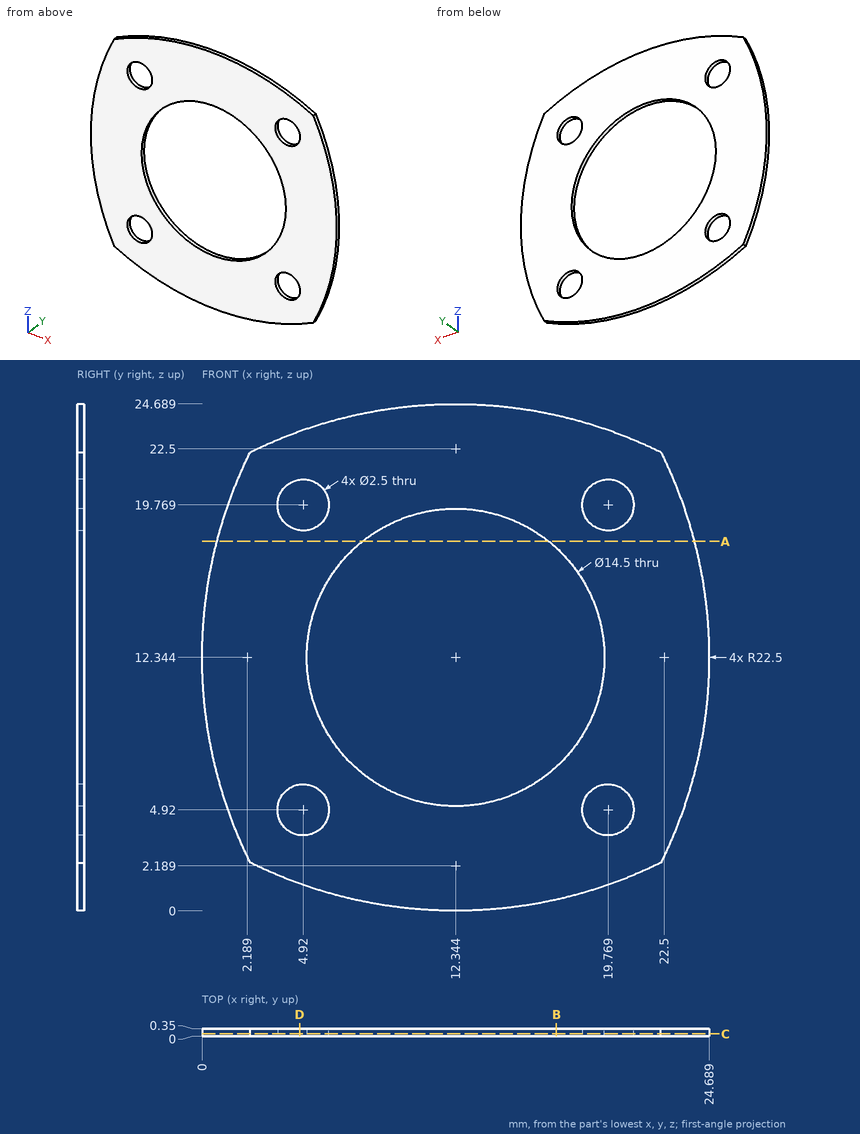
The figure shows three views and two pictorial views of one solid part (mm, origin at its lowest corner). Answer the questions. Round coordinates to 2 decimals unless told otherwise and drop trailing zeros. Write each loop counter-clockwise with the first axis right and the second up, starting at its lowest first coordinate (ties: lowest second). Pieces come first, ordered by that corner, then holes. Notation, with made-up numbers: (-28, -16) - (2, -16) arc R16 ccw to (2, 8) - close; hole circle Ø6 at (25, 82.25). An arc over 180 degrees is marked (long way). Answer in a Markdown table with one row per item. Add a question column.
1. Find the intervals of material crossed by line 1 along X through (y, z) = (0.25, 4) (1 decimal); line 2 along Z through (x, y) = (4.25, 0.15) (1 decimal), in increasing order. Write a range as from..to.
2. A cutting plane is placed at B-B, the plane x = 17.25. Determine the outline of the cut face in (y, z).
3. A cutting plane is placed at A-A, the plane z = 18. Determine the outline of the cut face in (x, y).
4. A cutting plane is placed at D-D, the plane x = 4.75. Determine the outline of the cut face in (y, z).
5. A cutting plane is placed at C-C, the plane y = 0.1. Count the separate pieces of the cut face and the enclosed holes in it, and give its area (3 significant figures).
Worked out:
| question | item | result |
|---|---|---|
| 1 | line 1 | 1.6..4.1, 5.8..18.9, 20.6..23.1 |
| 1 | line 2 | 1.5..3.9, 6..18.7, 20.8..23.2 |
| 2 | outline | (0, 0.54) - (0.35, 0.54) - (0.35, 7.01) - (0, 7.01) - close; (0, 17.68) - (0.35, 17.68) - (0.35, 24.15) - (0, 24.15) - close |
| 3 | outline | (0.72, 0) - (7.81, 0) - (7.81, 0.35) - (0.72, 0.35) - close; (16.88, 0) - (23.97, 0) - (23.97, 0.35) - (16.88, 0.35) - close |
| 4 | outline | (0, 1.32) - (0.35, 1.32) - (0.35, 3.68) - (0, 3.68) - close; (0, 6.16) - (0.35, 6.16) - (0.35, 18.53) - (0, 18.53) - close; (0, 21.01) - (0.35, 21.01) - (0.35, 23.37) - (0, 23.37) - close |
| 5 | separate pieces | 1 |
| 5 | enclosed holes | 5 |
| 5 | area | 342 mm^2 |
